Could you check a few things on this model? Use its own coordinates, in mm. A direction names the side the tool comes from. Coordinates: 2 decimals unless noted, no trailing zeros. Loops run counter-clockwise (first coordinate to the right, second up) from the corner with the lowest first, then second, coordinate; pieces in that order, holes last.
from build123d import *

# Parameters (mm, degrees)
F0_R     = 1.05
F1_DEPTH = 2
F2_DEPTH = 50
F3_COUNT = 6
F4_DEPTH = 50.001


with BuildPart() as f1:
    # F0 (on Top) → F1 (new body)
    with BuildSketch(Plane.XY):
        with BuildLine():
            Line((18.2298347497, 10.525), (19.918584287, 11.5))
            Line((19.918584287, 11.5), (0, 23))
            Line((0, 23), (0, 21.05))
            ThreePointArc((0, 21.05), (0.7424621202, 20.7424621202), (1.05, 20))
            ThreePointArc((1.05, 20), (0.7424621202, 19.2575378798), (0, 18.95))
            Line((0, 18.95), (0, 16.05))
            ThreePointArc((0, 16.05), (0.7424621202, 15.7424621202), (1.05, 15))
            ThreePointArc((1.05, 15), (0.7424621202, 14.2575378798), (0, 13.95))
            Line((0, 13.95), (0, 11.05))
            ThreePointArc((0, 11.05), (0.7424621202, 10.7424621202), (1.05, 10))
            ThreePointArc((1.05, 10), (0.7424621202, 9.2575378798), (0, 8.95))
            Line((0, 8.95), (0, 6.05))
            ThreePointArc((0, 6.05), (0.7424621202, 5.7424621202), (1.05, 5))
            ThreePointArc((1.05, 5), (0.7424621202, 4.2575378798), (0, 3.95))
            Line((0, 3.95), (0, 1.05))
            ThreePointArc((0, 1.05), (0.525, 0.909326674), (0.909326674, 0.525))
            Line((0.909326674, 0.525), (3.4208003449, 1.975))
            ThreePointArc((3.4208003449, 1.975), (3.8051270189, 3.409326674), (5.2394536929, 3.025))
            Line((5.2394536929, 3.025), (7.7509273639, 4.475))
            ThreePointArc((7.7509273639, 4.475), (8.1352540378, 5.909326674), (9.5695807118, 5.525))
            Line((9.5695807118, 5.525), (12.0810543828, 6.975))
            ThreePointArc((12.0810543828, 6.975), (12.4653810568, 8.409326674), (13.8997077307, 8.025))
            Line((13.8997077307, 8.025), (16.4111814017, 9.475))
            ThreePointArc((16.4111814017, 9.475), (16.7955080757, 10.909326674), (18.2298347497, 10.525))
        make_face()
        with Locations((4.3301270189, 7.5)):
            Circle(F0_R, mode=Mode.SUBTRACT)
        with Locations((4.3301270189, 12.5)):
            Circle(F0_R, mode=Mode.SUBTRACT)
        with Locations((8.6602540378, 10)):
            Circle(F0_R, mode=Mode.SUBTRACT)
        with Locations((12.9903810568, 12.5)):
            Circle(F0_R, mode=Mode.SUBTRACT)
        with Locations((4.3301270189, 17.5)):
            Circle(F0_R, mode=Mode.SUBTRACT)
        with Locations((8.6602540378, 15)):
            Circle(F0_R, mode=Mode.SUBTRACT)
        with BuildLine():
            Line((0, 0), (0.909326674, 0.525))
            ThreePointArc((0.909326674, 0.525), (0.525, 0.909326674), (0, 1.05))
            Line((0, 1.05), (0, 0))
        make_face()
    extrude(amount=F1_DEPTH)

    # F0 (on Top) → F2 (join)
    with BuildSketch(Plane.XY):
        with BuildLine():
            Line((0, 25.3094010768), (0, 23))
            ThreePointArc((0, 23), (2.4761009674, 22.8663272958), (4.9234204468, 22.4668629564))
            Line((4.9234204468, 22.4668629564), (0, 25.3094010768))
        make_face()
        with BuildLine():
            ThreePointArc((16.9951638402, 15.4972386587), (18.5647698457, 13.577529988), (19.918584287, 11.5))
            Line((19.918584287, 11.5), (21.918584287, 12.6547005384))
            Line((21.918584287, 12.6547005384), (16.9951638402, 15.4972386587))
        make_face()
        with BuildLine():
            Line((0, 23), (19.918584287, 11.5))
            ThreePointArc((19.918584287, 11.5), (18.5647698457, 13.577529988), (16.9951638402, 15.4972386587))
            Line((16.9951638402, 15.4972386587), (4.9234204468, 22.4668629564))
            ThreePointArc((4.9234204468, 22.4668629564), (2.4761009674, 22.8663272958), (0, 23))
        make_face()
    extrude(amount=F2_DEPTH)

    # F3: F1 ×6 about axis
    f3_axis = Axis((0, 0, 1), (0, 0, -1))


with BuildPart() as f1_1:
    add(f1.part)
    for i in range(1, F3_COUNT):
        add(f1.part.rotate(f3_axis, i * 360 / F3_COUNT))

    # F0 (on Top) → F4 (cut, through all)
    with BuildSketch(Plane.XY):
        with BuildLine():
            ThreePointArc((1.05, 0), (1.0142221176, 0.2717599974), (0.909326674, 0.525))
            Line((0.909326674, 0.525), (0, 0))
            Line((0, 0), (0, 1.05))
            ThreePointArc((0, 1.05), (-0.7424621202, -0.7424621202), (1.05, 0))
        make_face()
        with BuildLine():
            Line((0, 0), (0.909326674, 0.525))
            ThreePointArc((0.909326674, 0.525), (0.525, 0.909326674), (0, 1.05))
            Line((0, 1.05), (0, 0))
        make_face()
    extrude(amount=F4_DEPTH, mode=Mode.SUBTRACT)


solid = f1_1.part
(1) Which directions (+Z, -Z, +X, -X, +Y, -Y) give clear straight access to the entire face, cutting with the end or side of a thin tool? Please do faces 1 (the face through (4.19, -16.46, 0.99)), 2 (the face through (-10.1, 17.17, 25.66)).
Answers:
face 1: +Z, -Z
face 2: +Z
(2) Imagine slicing it at C-C, the plane x = 15. Write out the boundary of the cut face in (y, z), and give its area (3 significant figures).
Answers:
outline: (-16.65, 0) - (16.65, 0) - (16.65, 50) - (14.34, 50) - (14.34, 2) - (-14.34, 2) - (-14.34, 50) - (-16.65, 50) - close
area: 288 mm2
(3) For pin 1 (2 mm diameter, centred on x = 12, z = 18.5, fed in from +Y); pin 2 (4 mm diameter, centred on x = -8.5, z = 39, fed in from +Y); pin 3 (6 mm diameter, centred on x = 0.5, y = 11.5, fed in from +Z), each with a flat end and sliding along its axis, tell me the tip position at first contact or that it passes through.
Answers:
pin 1: stops at y = 18.96
pin 2: stops at y = 21.56
pin 3: stops at z = 2
(4) Imagine slicing it at A-A, the plane z = 28.5. Write out the boundary of the cut face in (x, y).
Answers:
outline: (-21.92, -12.65) - (0, -25.31) - (21.92, -12.65) - (21.92, 12.65) - (0, 25.31) - (-21.92, 12.65) - close; hole (-19.92, -11.5) - (0, -23) - (19.92, -11.5) - (19.92, 11.5) - (0, 23) - (-19.92, 11.5) - close
(5) I need wall thicknesses on probe 1 along X at (y, z) = (-5, 33); probe 2 along Y at (x, z) = (-10, 39); probe 3 along Y at (x, z) = (-4, 4). Which ranges of each line are inside material? Lowest first, please.
Answers:
probe 1: x = -21.92 to -19.92, 19.92 to 21.92
probe 2: y = -19.54 to -17.23, 17.23 to 19.54
probe 3: y = -23 to -20.69, 20.69 to 23
(6) Imagine slicing it at B-B, the plane y = -17.5. Write out the boundary of the cut face in (x, z).
Answers:
outline: (-13.53, 0) - (-5.38, 0) - (-5.38, 2) - (-9.53, 2) - (-9.53, 50) - (-13.53, 50) - close; (-3.28, 0) - (3.28, 0) - (3.28, 2) - (-3.28, 2) - close; (5.38, 0) - (13.53, 0) - (13.53, 50) - (9.53, 50) - (9.53, 2) - (5.38, 2) - close
